from build123d import *

# Parameters (mm, degrees)
SKETCH_1_W          = 130
SKETCH_1_H          = 60
SKETCH_1_R          = 1.5
EXTRUDE_1_DEPTH     = 3
SKETCH_2_R          = 1.5
CUT_EXTRUDE_1_DEPTH = 72.651936471
CUT_EXTRUDE_2_DEPTH = 72.651936471
FILLET_1_R          = 2


with BuildPart() as part:
    # 草图1 → 凸台-拉伸1 (new body)
    with BuildSketch(Plane(origin=(0, 0, 0), x_dir=(1, 0, 0), z_dir=(0, 1, 0))):
        Rectangle(SKETCH_1_W, SKETCH_1_H)
        with Locations(Location((-60, 10, 0), (0, 0, 270))):
            Circle(SKETCH_1_R, mode=Mode.SUBTRACT)
        with Locations(Location((-60, -10, 0), (0, 0, 270))):
            Circle(SKETCH_1_R, mode=Mode.SUBTRACT)
    extrude(amount=EXTRUDE_1_DEPTH)

    # 草图2 → 切除-拉伸1 (cut, through all)
    with BuildSketch(Plane(origin=(0, 3, 0), x_dir=(1, 0, 0), z_dir=(0, 1, 0))):
        with Locations(Location((-30, 24, 0), (0, 0, 270))):
            Circle(SKETCH_2_R)
        with Locations(Location((-50, 24, 0), (0, 0, 270))):
            Circle(SKETCH_2_R)
        with Locations(Location((-50, -24, 0), (0, 0, 90))):
            Circle(SKETCH_2_R)
        with Locations(Location((-30, -24, 0), (0, 0, 90))):
            Circle(SKETCH_2_R)
    extrude(amount=-CUT_EXTRUDE_1_DEPTH, mode=Mode.SUBTRACT)

    # 草图3 → 切除-拉伸2 (cut, through all)
    with BuildSketch(Plane(origin=(0, 3, 0), x_dir=(1, 0, 0), z_dir=(0, 1, 0))):
        Polygon((-55, 0), (-40, 15), (-40, 5), (55, 5), (55, -5), (-40, -5), (-40, -15), align=None)
        Polygon((-15, 25), (55, 25), (55, 15), (-25, 15), align=None)
        Polygon((55, -15), (-25, -15), (-15, -25), (55, -25), align=None)
    extrude(amount=-CUT_EXTRUDE_2_DEPTH, mode=Mode.SUBTRACT)

    # 圆角1
    fillet_1_edges = [part.edges().sort_by_distance(p)[0] for p in [
        (55, 1.5, 15),
        (55, 1.5, 25),
        (-15, 1.5, 25),
        (-25, 1.5, 15),
        (-25, 1.5, -15),
        (-15, 1.5, -25),
        (55, 1.5, -25),
        (55, 1.5, -15),
        (-40, 1.5, 15),
        (-55, 1.5, 0),
        (-40, 1.5, -15),
        (-40, 1.5, -5),
        (55, 1.5, -5),
        (55, 1.5, 5),
        (-40, 1.5, 5),
        (65, 1.5, 30),
        (-65, 1.5, 30),
        (-65, 1.5, -30),
        (65, 1.5, -30),
    ]]
    fillet(fillet_1_edges, radius=FILLET_1_R)


solid = part.part
Geometry: final body of the model. Coordinates: model frame, mm. A direction names the side the tool comes from. Round coordinates to 2 decimals unless told otherwise and drop trailing zeros. Loops run counter-clockwise (first coordinate to the right, second up) from the corner with the lowest first, then second, coordinate; pieces in that order, holes last. Notation, with made-up numbers: M 72.5,11 L 84.5,11 A30 cw 84.5,43 Z; hole C 86,3.25 d10. An arc over 180 degrees is marked long. Put each result on its own line as item: value. Start each with the question number.
(1) Section query C-C (y = 0.5). State how many separate pieces and enclosed holes the cut face has, then the cut area to 3 significant figures.
(2) Material intervals for line 1 along Z through (x, y) = (28, 1.25); line 2 along X through (y, z) = (1.4, 10); line 3 along X through (y, z) = (1.15, -24), sorted ascending. Write a range as [from, to].
(3) Draft query along X for faces 3 (the face through (-48, 2, 7)), 4 (the face through (-1, 3, -7)). Return one class per face: +X half, -X half, draft (parallel to the pull), parting line (faces both ways), or undercut.
(4) Set-up query: faces 1 (the face through (17, 2, 15)), 2 (the face through (-1, 1, 30)). Return all of +Z, -Z, +X, -X, +Y, -Y with unobstructed straight access to the full face (end or side cutting, diameter ignored); none if empty.
(5) Section query A-A (x = 36.5). Return loops of the section in (y, z).
(6) Section query B-B (x = -30). Return loops of the section in (y, z).
Findings below:
1. separate pieces: 1
1. enclosed holes: 9
1. area: 5,100 mm2
2. line 1: z = [-30, -25], [-15, -5], [5, 15], [25, 30]
2. line 2: x = [-65, -61.5], [-58.5, -45], [-40, 65]
2. line 3: x = [-65, -51.5], [-48.5, -31.5], [-28.5, -16], [54.73, 65]
3. face 3: undercut
3. face 4: draft
4. face 1: +Y, -Y
4. face 2: +Z, +X, -X, +Y, -Y
5. outline: M 0,-30 L 3,-30 L 3,-25 L 0,-25 Z; M 0,-15 L 3,-15 L 3,-5 L 0,-5 Z; M 0,5 L 3,5 L 3,15 L 0,15 Z; M 0,25 L 3,25 L 3,30 L 0,30 Z
6. outline: M 0,-30 L 3,-30 L 3,-25.5 L 0,-25.5 Z; M 0,-22.5 L 3,-22.5 L 3,-5 L 0,-5 Z; M 0,5 L 3,5 L 3,22.5 L 0,22.5 Z; M 0,25.5 L 3,25.5 L 3,30 L 0,30 Z
